Build history of the part. All positions in model axes, mm. A direction names the side the tool comes from. Coordinates: 2 decimals unless noted, no trailing zeros. Write each loop counter-clockwise with the first axis right and the second up, starting at its lowest first coordinate (ties: lowest second). Pieces come first, ordered by that corner, then holes. Notation, with made-up numbers: M -0.75,-13 L 37.25,-13 A8 cw 37.25,-5 Z; hole C -30,-10.5 d8. An arc over 180 degrees is marked long. Use CSV: the item, a comma, the result in double quotes. Start each with the question number.
Autodesk Inventor part; units mm, degrees
ref_plane "YZ Plane" through (0, 0, 0) normal (1, 0, 0) x (0, 1, 0)
ref_plane "XZ Plane" through (0, 0, 0) normal (0, 1, 0) x (-1, 0, 0)
ref_plane "XY Plane" through (0, 0, 0) normal (0, 0, 1) x (1, 0, 0)
sketch "Sketch1" plane through (0, 0, 0) normal (0, 1, 0) x (-1, 0, 0)
  line L0 (-35.3568, 82.55) -> (35.3568, 82.55)
  line L1 (35.3568, 82.55) -> (35.3568, -82.55)
  line L2 (35.3568, -82.55) -> (-35.3568, -82.55)
  line L3 (-35.3568, 82.55) -> (35.3568, -82.55) construction
  line L4 (35.3568, 82.55) -> (-35.3568, -82.55) construction
  line L5 (-35.3568, 88.9) -> (42.3418, 88.9)
  line L6 (42.3418, 88.9) -> (42.3418, -88.9)
  line L7 (42.3418, -88.9) -> (-35.3568, -88.9)
  line L8 (42.3418, 88.9) -> (-35.3568, -88.9) construction
  line L9 (42.3418, -88.9) -> (-35.3568, 88.9) construction
  line L10 (3.4925, 0) -> (42.3418, 0) construction
  line L11 (-35.3568, -88.9) -> (-35.3568, -82.55)
  line L12 (-35.3568, 82.55) -> (-35.3568, 88.9)
  point P0 (0, 0)
  point P1 (35.3568, 0)
  dimension "d1" = 165.1
  dimension "d2" = 177.8
  dimension "d3" = 77.6986
  dimension "d4" = 70.7136
  dimension "d5" = 70.7136
extrude "Extrusion1" add sketch "Sketch1" along normal blind 25.4
properties part number "BoxHolders"
1. Flat gauge pin, fed straight in: pin 1 (12.5 mm diameter, centred on y = 15.5, z = -27, fed in from +X). Where does the tip first touch, or does it go through?
2. Slice it at A-A (x = 12). List the corners of the cut face in (y, z).
3. Drill centre lines: line 1 along Z through (x, y) = (-10, 4); line 2 along X through (y, z) = (6, -35.5). Where is each one in solid material? Low to high. Write a range as from..to.
4. 3-axis set-ups, long thin cutter, end or side, ignore diameter. For faces 4 (the flat face through (35.357, 13, -86)), 5 (the flat face through (0, 13, 82.55)): which of +Z, -Z, +X, -X, +Y, -Y reach the whole face in a straight line?
5. Slice it at C-C (z = 22). List the corners of the cut face in (x, y), and give its area (3 significant figures).
6. Pull direction Z, two halves, no side cores. Call faces 1 (the flat face through (0, 13, -82.55)), 2 (the flat face through (-3, 13, 88.9)), 3 (the flat face through (-42.342, 13, 1)): pulls with the +Z half, pulls with the -Z half, needs draft (parallel to the pull), parting line crosses it, or undercut.
7. Slice it at B-B (y = 8.5). List the corners of the cut face in (x, z), and give its area (3 significant figures).
Established:
1,pin 1,"stops at x = -35.36"
2,outline,"M 0,-88.9 L 25.4,-88.9 L 25.4,-82.55 L 0,-82.55 Z; M 0,82.55 L 25.4,82.55 L 25.4,88.9 L 0,88.9 Z"
3,line 1,"z = -88.9..-82.55, 82.55..88.9"
3,line 2,"x = -42.34..-35.36"
4,face 4,"+Z, -Z, +X, +Y, -Y"
4,face 5,"+X, +Y, -Y"
5,outline,"M -42.34,0 L -35.36,0 L -35.36,25.4 L -42.34,25.4 Z"
5,area,"177 mm2"
6,face 1,"undercut"
6,face 2,"pulls with the +Z half"
6,face 3,"needs draft"
7,outline,"M -42.34,-88.9 L 35.36,-88.9 L 35.36,-82.55 L -35.36,-82.55 L -35.36,82.55 L 35.36,82.55 L 35.36,88.9 L -42.34,88.9 Z"
7,area,"2,140 mm2"
